from build123d import *

# Parameters (mm, degrees)
F1_DEPTH = 10


with BuildPart() as f1:
    # F0 (on Top) → F1 (new body)
    with BuildSketch(Plane.XY):
        with BuildLine():
            Line((28.628895, 12), (28.628895, 0))
            Line((28.628895, 0), (78.628895, 0))
            Line((78.628895, 0), (78.628895, 50))
            Line((78.628895, 50), (3.628895, 50))
            Line((3.628895, 50), (3.628895, 34))
            Line((3.628895, 34), (28.628895, 34))
            ThreePointArc((28.628895, 34), (39.628895, 23), (28.628895, 12))
        make_face()
    extrude(amount=F1_DEPTH)


solid = f1.part
Read the model definition and answer for the solid it produces. Units are mm, in the model's axes. A direction names the side the tool comes from. Give positions to 0.01 mm unless a question says otherwise; leave off trailing zeros. Write each loop counter-clockwise with the first axis right and the second up, starting at its lowest first coordinate (ties: lowest second). Pieces come first, ordered by that corner, then holes. Notation, with made-up numbers: (48.5, 87.5) - (76.5, 87.5) arc R30 ccw to (76.5, 122.5) - close; hole circle Ø3 at (34.5, -31.5). An arc over 180 degrees is marked (long way). Return JSON: item names as keys, results as strings.
Q1. For a pull along Y with two mould halves and no side action, classify faces 3 (the face through (42, 50, 5)), 4 (the face through (39.626, 23.242, 4.93)), 5 (the face through (28.629, 6, 5)) as released by +Y, released by -Y, zero draft, split by the parting line, or undercut.
Reply:
{"face 3": "released by +Y", "face 4": "undercut", "face 5": "zero draft"}
Q2. A cutting plane is placed at A-A, the plane z = 6.5. Determine the outline of the cut face in (x, y), and give its area (3 significant figures).
Reply:
{"outline": "(3.63, 34) - (28.63, 34) arc R11 cw to (28.63, 12) - (28.63, 0) - (78.63, 0) - (78.63, 50) - (3.63, 50) - close", "area": "2,710 mm²"}
Q3. A cutting plane is placed at B-B, the plane y = 23. Determine the outline of the cut face in (x, z), and give its area (3 significant figures).
Reply:
{"outline": "(39.63, 0) - (78.63, 0) - (78.63, 10) - (39.63, 10) - close", "area": "390 mm²"}
Q4. A cutting plane is placed at C-C, the plane x = 24.5. Determine the outline of the cut face in (y, z).
Reply:
{"outline": "(34, 0) - (50, 0) - (50, 10) - (34, 10) - close"}
Q5. Given P1, Ø5, axis at y = 7, z = 8, coming from the -X side; P2, Ø6, axis at y = 22, z = 3, coming from the -X side; P3, Ø1.5, axis at x = 14.5, y = 44, coming from the -Z side; P4, Ø1.5, axis at y = 21, z = 1.5, coming from the -X side, each flat-ended and moving along its own axis, determine where each tip first touches the part or whether it passes through.
Reply:
{"P1": "x = 28.63", "P2": "x = 38.88", "P3": "z = 0", "P4": "x = 39.28"}
Q6. Consider line 1 along X through (y, z) = (11, 8.5); line 2 along Y through (x, z) = (25.5, 6); line 3 along Y through (x, z) = (36.5, 6.5). Determine where each line is inside the solid, lowest interval first. Write a range as [from, to].
Reply:
{"line 1": "[28.63, 78.63]", "line 2": "[34, 50]", "line 3": "[0, 15.32], [30.68, 50]"}
Q7. For faces 1 (the face through (16, 34, 5)), 2 (the face through (49, 25, 10)), determine the directions among +Z, -Z, +X, -X, +Y, -Y from which every point of the face is accessible in a straight line to the end or side of a thin tool.
Reply:
{"face 1": "+Z, -Z, -X, -Y", "face 2": "+Z, +X, -X, +Y, -Y"}
